from build123d import *

# Parameters (mm, degrees)
SKETCH1_W           = 12
SKETCH1_H           = 24
BOSS_EXTRUDE1_DEPTH = 5.5
SKETCH2_W           = 2
SKETCH2_H           = 24
BOSS_EXTRUDE2_DEPTH = 29.5
BOSS_EXTRUDE4_START = 3
SKETCH4_W           = 5.5
SKETCH4_H           = 24
BOSS_EXTRUDE4_DEPTH = 18
SKETCH5_W           = 9.25
SKETCH5_H           = 18
CUT_EXTRUDE1_DEPTH  = 1.5
FILLET1_R           = 2.5
SKETCH6_R           = 2
SKETCH6_R_2         = 1.5
CUT_EXTRUDE2_DEPTH  = 31.170349683
FILLET2_R           = 1.5


with BuildPart() as part:
    # Sketch1 → Boss-Extrude1 (new body)
    with BuildSketch(Plane(origin=(0, 0, 0), x_dir=(1, 0, 0), z_dir=(0, 1, 0))):
        Rectangle(SKETCH1_W, SKETCH1_H)
    extrude(amount=BOSS_EXTRUDE1_DEPTH)

    # Sketch2 → Boss-Extrude2 (add)
    with BuildSketch(Plane(origin=(0, 0, 0), x_dir=(1, 0, 0), z_dir=(0, 1, 0))):
        with Locations((7, 0)):
            Rectangle(SKETCH2_W, SKETCH2_H)
    extrude(amount=BOSS_EXTRUDE2_DEPTH)

    # Sketch4 → Boss-Extrude4 (add)
    with BuildSketch(Plane(origin=(0, 5.5, 0), x_dir=(1, 0, 0), z_dir=(0, 1, 0)).offset(BOSS_EXTRUDE4_START)):
        with Locations((3.25, 0)):
            Rectangle(SKETCH4_W, SKETCH4_H)
    extrude(amount=BOSS_EXTRUDE4_DEPTH)

    # Sketch5 → Cut-Extrude1 (cut)
    with BuildSketch(Plane.ZY.offset(-0.5)):
        with Locations((0, 17.5)):
            Rectangle(SKETCH5_W, SKETCH5_H)
    extrude(amount=-CUT_EXTRUDE1_DEPTH, mode=Mode.SUBTRACT)

    # Fillet1
    # the kernel refuses this fillet: 2.5 mm, written as the material it takes off along each edge
    with BuildSketch(Plane(origin=(0.5, 32.228219619, 4.625), x_dir=(0, 0, 1), z_dir=(0, -1, 0)), Plane(origin=(0.5, 8.5, -4.625), x_dir=(0, 0, -1), z_dir=(0, 1, 0))) as fillet1_piece_1:
        with BuildLine():
            CenterArc((2.291287847, -2.5), FILLET1_R, 90, 66.421821522)
            Line((0, -1.5), (0, 0))
            Line((0, 0), (2.291287847, 0))
        make_face()
    extrude(amount=23.728219619, mode=Mode.SUBTRACT)

    # Sketch6 → Cut-Extrude2 (cut, through all)
    with BuildSketch(Plane(origin=(0, 26.5, 0), x_dir=(1, 0, 0), z_dir=(0, 1, 0))):
        with Locations(Location((3, -6, 0), (0, 0, 270))):
            Circle(SKETCH6_R)
        with Locations(Location((3, 6, 0), (0, 0, 90))):
            Circle(SKETCH6_R)
        with Locations(Location((3, 0, 0), (0, 0, 270))):
            Circle(SKETCH6_R_2)
    extrude(amount=-CUT_EXTRUDE2_DEPTH, mode=Mode.SUBTRACT)

    # Fillet2
    fillet2_edges = [part.edges().sort_by_distance(p)[0] for p in [
        (0.5, 17.5, -12),
        (0.5, 17.5, 12),
    ]]
    fillet(fillet2_edges, radius=FILLET2_R)


solid = part.part
The model under review builds one solid part; all positions refer to its coordinate system, in mm. A direction names the side the tool comes from. Give positions to 0.01 mm unless a question says otherwise; leave off trailing zeros. Loops run counter-clockwise (first coordinate to the right, second up) from the corner with the lowest first, then second, coordinate; pieces in that order, holes last. Notation, with made-up numbers: (21.5, 58.25) -> (26.5, 58.25) arc R25 cw to (26.5, 70.25) -> close; hole circle Ø3 at (25, 24). An arc over 180 degrees is marked (long way). Answer as a JSON object with one key per item and string values. Group by question number.
Q1. Take a section at D-D (x = 3). State how many separate pieces and enclosed holes the cut face has, plus the area to 4 significant figures.
Q2. Wall thickness on line 1 along Z through (x, y) = (3, 21.25); line 2 along X through (y, z) = (2.8, 6); line 3 along Y through (x, z) = (-3.75, 10.5): over which ranges is each line inside the solid? List them lowest first.
Q3. Take a section at C-C (z = -2.25). Write out the cut boundary in (x, y).
Q4. Tool access review of faces 5 (the flat face through (5, 8.5, 0)), 6 (the cylindrical face through (0.665, 17.374, -6.024)), 7 (the flat face through (0.5, 17, 9)), 8 (the cylindrical face through (0.93, 17.63, -11.55)): name each direction out of +Z, -Z, +X, -X, +Y, -Y from which nothing blocks a thin tool from reaching the whole face with its end or side.
Q5. Draft analysis for pull direction X (two halves, no side actions). For faces 1 (the flat face through (8, 15, 0)), 2 (the flat face through (2.5, 11.3, -12)), 3 (the cylindrical face through (4.45, 17.63, 7.38)), 4 (the flat face through (-6, 3, 0)), state which applies: pulls with the +X half, pulls with the -X half, needs draft (parallel to the pull), parting line crosses it, or undercut.
Q6. Insertion check: pin 1 (2.5 mm diameter, centred on x = 3, z = 6, fed in from +Y); pin 2 (4.5 mm diameter, centred on x = 4, z = 4.5, fed in from +Y); pin 3 (1.1 mm diameter, centred on y = 22, z = 9, fed in from -X); pin 4 (3.5 mm diameter, centred on y = 14, z = -2.5, fed in from -X). Each pin has a flat end and moves straight along its axis. Give the tip position at first contact, or say it passes through.
Q7. Take a section at A-A (y = 4.5). Write out the cut boundary in (x, z).
Q8. Take a section at B-B (x = 5.5). Write out the cut boundary in (y, z), plus the area to 3 significant figures.
Answer below:
{
 "1": {"separate pieces": "8", "enclosed holes": "0", "area": "305.5 mm2"},
 "2": {"line 1": "z = -12 to -8, -4 to -1.5, 1.5 to 4, 8 to 12", "line 2": "x = -6 to 1, 5 to 8", "line 3": "y = 0 to 5.5"},
 "3": {"outline": "(-6, 0) -> (8, 0) -> (8, 29.5) -> (6, 29.5) -> (6, 26.5) -> (2, 26.5) -> (2, 8.5) -> (6, 8.5) -> (6, 5.5) -> (-6, 5.5) -> close"},
 "4": {"face 5": "+Z, -Z, -X", "face 6": "-X, +Y", "face 7": "+Z, -Z, -X, +Y", "face 8": "-Z, -X, +Y"},
 "5": {"face 1": "pulls with the +X half", "face 2": "needs draft", "face 3": "undercut", "face 4": "pulls with the -X half"},
 "6": {"pin 1": "passes through", "pin 2": "stops at y = 29.5", "pin 3": "stops at x = 0.5", "pin 4": "stops at x = 2"},
 "7": {"outline": "(-6, -12) -> (8, -12) -> (8, 12) -> (-6, 12) -> close; hole circle Ø4 at (3, -6); hole circle Ø4 at (3, 6); hole circle Ø3 at (3, 0)"},
 "8": {"outline": "(0, -12) -> (5.5, -12) -> (5.5, 12) -> (0, 12) -> close; (8.5, -12) -> (26.5, -12) -> (26.5, 12) -> (8.5, 12) -> close", "area": "564 mm2"}
}
